```python
from build123d import *

# Parameters (mm, degrees)
SKETCH1_R           = 4.05765
SKETCH1_R_2         = 3.5306
SKETCH1_R_3         = 2.032
SKETCH1_R_4         = 1.6002
BOSS_EXTRUDE1_DEPTH = 3.175
SKETCH1_7_R         = 1.6002
CUT_EXTRUDE4_DEPTH  = 0.9525
SKETCH3_W           = 1.27
SKETCH3_H           = 1.905
FILLET1_R           = 0.635
FILLET2_R           = 0.635


with BuildPart() as part:
    # Sketch1 → Boss-Extrude1 (new, symmetric)
    with BuildSketch(Plane.XY):
        with BuildLine():
            Line((9.525, 38.1), (9.525, 0))
            ThreePointArc((9.525, 0), (0, -9.525), (-9.525, 0))
            Line((-9.525, 0), (-9.525, 38.1))
            Line((-9.525, 38.1), (9.525, 38.1))
        make_face()
        Circle(SKETCH1_R, mode=Mode.SUBTRACT)
        with Locations((0, 19.05)):
            Circle(SKETCH1_R_2, mode=Mode.SUBTRACT)
        with Locations((-6.35, 32.004)):
            Circle(SKETCH1_R_3, mode=Mode.SUBTRACT)
        with Locations((6.35, 32.004)):
            Circle(SKETCH1_R_3, mode=Mode.SUBTRACT)
        with Locations((6.985, 9.525)):
            Circle(SKETCH1_R_4, mode=Mode.SUBTRACT)
    extrude(amount=BOSS_EXTRUDE1_DEPTH, both=True)

    # Sketch1<7> → Cut-Extrude4 (cut, symmetric)
    with BuildSketch(Plane.XY):
        with BuildLine():
            Line((9.525, 6.6548), (9.525, 12.3952))
            Line((9.525, 12.3952), (6.985, 12.3952))
            ThreePointArc((6.985, 12.3952), (4.1148, 9.525), (6.985, 6.6548))
            Line((6.985, 6.6548), (9.525, 6.6548))
        make_face()
        with Locations((6.985, 9.525)):
            Circle(SKETCH1_7_R, mode=Mode.SUBTRACT)
    extrude(amount=CUT_EXTRUDE4_DEPTH, both=True, mode=Mode.SUBTRACT)

    # Cut-Sweep1: sweep along a path in Sketch2
    with BuildLine(Plane.XY.offset(3.175)) as cut_sweep1_path:
        Line((9.525, 6.6548), (9.525, 0))
        ThreePointArc((9.525, 0), (0, -9.525), (-9.525, 0))
        Line((-9.525, 0), (-9.525, 6.35))
    # Sketch3 → Cut-Sweep1 (sweep, cut)
    with BuildSketch(Plane(origin=(0, 6.6548, 0), x_dir=(1, 0, 0), z_dir=(0, 1, 0))):
        with Locations((8.89, 0)):
            Rectangle(SKETCH3_W, SKETCH3_H)
    sweep(path=cut_sweep1_path.line, mode=Mode.SUBTRACT)

    # Fillet1
    fillet1_edges = [part.edges().sort_by_distance(p)[0] for p in [
        (0, -9.525, 3.175),
        (-9.525, 19.05, -3.175),
        (0, 38.1, -3.175),
        (9.525, 19.05, 3.175),
        (9.525, 19.05, -3.175),
        (0, -9.525, -3.175),
        (-9.525, 38.1, 0),
        (9.525, 38.1, 0),
        (0, 38.1, 3.175),
        (-9.525, 19.05, 3.175),
    ]]
    fillet(fillet1_edges, radius=FILLET1_R)

    # Fillet2
    fillet2_edges = [part.edges().sort_by_distance(p)[0] for p in [
        (8.255, 6.6548, 0),
        (9.525, 12.3952, 0),
        (-9.525, 6.35, 0),
        (-8.255, 6.35, 0),
    ]]
    fillet(fillet2_edges, radius=FILLET2_R - 0.0001)  # a hair under: the kernel refuses the full size


solid = part.part
```
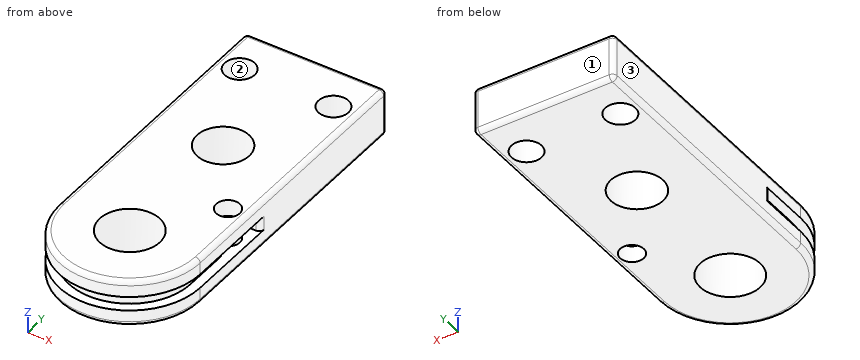
Geometry check sheet. Reference: the model listing, model coordinates, mm. Face numbers are marked on the shaded views. Coordinates: 2 decimals unless noted, no trailing zeros. Write each loop counter-clockwise with the first axis right and the second up, starting at its lowest first coordinate (ties: lowest second). Pieces come first, ordered by that corner, then holes. Notation, with made-up numbers: M 73.5,84 L 107.5,84 A19 cw 107.5,100 Z; hole C 89,-0.5 d4. An arc over 180 degrees is marked long. One line per item, written item: value. Start each with the question number.
(1) Sectioned sample at B-B, the plane y = 8.5. Enter the section's corners in (x, z) (1 decimal), and give its area (3 significant figures).
(2) Sectioned sample at C-C, the plane z = 1.5. Enter the section's corners in (x, y) (3 decimals), and give its area (3 significant figures).
(3) Sectioned sample at D-D, the plane y = 31. Enter the section's corners in (x, z) (3 decimals), and give its area (3 significant figures).
(4) Sectioned sample at A-A, the plane x = 0. Enter the section's corners in (y, z) (1 decimal).
(5) Depth check by flat-ended pin: pin 1 (3 mm diameter, centred on x = 4, z = 2, fed in from -Y); pin 2 (1.5 mm diameter, centred on x = -6.5, z = -1, fed in from -Y). Enter the tip coordinate at first touch or a pass-through.
(6) Release check for a two-part mould opening along Y. For the marked faces 1, 2 and 3 record: released by +Y, released by -Y, zero draft, split by the parting line, or undercut.
(7) Scan lines: line 1 along Y through (x, z) = (0, -0.5) (3 decimals); line 2 along Y through (x, z) = (0.5, 1.5); line 3 along X through (y, z) = (33.5, 1.5) (3 decimals). Record each from-to range of solid material in increasing order. Write a range as [from, to].
Filled sheet:
1. outline: M -9.5,-2.5 A0.6 ccw -8.9,-3.2 L 5.8,-3.2 L 5.8,-1 L 4.3,-1 L 4.3,1 L 5.8,1 L 5.8,3.2 L -8.9,3.2 A0.6 ccw -9.5,2.5 Z; M 8.2,-3.2 L 8.9,-3.2 A0.6 ccw 9.5,-2.5 L 9.5,-1 L 8.2,-1 Z; M 8.2,1 L 9.5,1 L 9.5,2.5 A0.6 ccw 8.9,3.2 L 8.2,3.2 Z
1. area: 99.8 mm²
2. outline: M -9.525,0 A9.525 ccw 9.525,0 L 9.525,37.465 A0.635 ccw 8.89,38.1 L -8.89,38.1 A0.635 ccw -9.525,37.465 Z; hole C -6.35,32.004 d4.064; hole C 0,0 d8.115; hole C 0,19.05 d7.061; hole C 6.35,32.004 d4.064; hole C 6.985,9.525 d3.2
2. area: 743 mm²
3. outline: M -9.525,-2.54 A0.635 ccw -8.89,-3.175 L -8.117,-3.175 L -8.117,3.175 L -8.89,3.175 A0.635 ccw -9.525,2.54 Z; M -4.583,-3.175 L 4.583,-3.175 L 4.583,3.175 L -4.583,3.175 Z; M 8.117,-3.175 L 8.89,-3.175 A0.635 ccw 9.525,-2.54 L 9.525,2.54 A0.635 ccw 8.89,3.175 L 8.117,3.175 Z
3. area: 75.7 mm²
4. outline: M -9.5,-2.5 A0.6 ccw -8.9,-3.2 L -4.1,-3.2 L -4.1,3.2 L -8.9,3.2 A0.6 ccw -9.5,2.5 L -9.5,1 L -8.3,1 L -8.3,-1 L -9.5,-1 Z; M 4.1,-3.2 L 15.5,-3.2 L 15.5,3.2 L 4.1,3.2 Z; M 22.6,-3.2 L 37.5,-3.2 A0.6 ccw 38.1,-2.5 L 38.1,2.5 A0.6 ccw 37.5,3.2 L 22.6,3.2 Z
5. pin 1: y = -9.19
5. pin 2: y = -7.59
6. face 1: released by +Y
6. face 2: undercut
6. face 3: zero draft
7. line 1: [-8.255, -4.058], [4.058, 15.519], [22.581, 38.1]
7. line 2: [-9.51, -4.03], [4.03, 15.55], [22.55, 38.1]
7. line 3: [-9.525, -7.725], [-4.975, 4.975], [7.725, 9.525]
